```python
from build123d import *

# Parameters (mm, degrees)
F0_R     = 2.032
F1_DEPTH = 19.05
F3_DEPTH = 304.8


with BuildPart() as f1:
    # F0 (on Top) → F1 (new body)
    with BuildSketch(Plane.XY):
        with BuildLine():
            Line((111.125, 152.4), (-69.85, 152.4))
            ThreePointArc((-69.85, 152.4), (-81.939168, 123.214168), (-111.125, 111.125))
            Line((-111.125, 111.125), (-111.125, -111.125))
            ThreePointArc((-111.125, -111.125), (-81.939168, -123.214168), (-69.85, -152.4))
            Line((-69.85, -152.4), (111.125, -152.4))
            Line((111.125, -152.4), (111.125, 152.4))
        make_face()
        with Locations((-63.5, -101.6)):
            Circle(F0_R, mode=Mode.SUBTRACT)
        with Locations((9.525, -127)):
            Circle(F0_R, mode=Mode.SUBTRACT)
        with Locations((77.7875, -101.6)):
            Circle(F0_R, mode=Mode.SUBTRACT)
        with Locations((-63.5, 101.6)):
            Circle(F0_R, mode=Mode.SUBTRACT)
        with Locations((9.525, 127)):
            Circle(F0_R, mode=Mode.SUBTRACT)
        with Locations((77.7875, 101.6)):
            Circle(F0_R, mode=Mode.SUBTRACT)
    extrude(amount=F1_DEPTH)

    # F2 (on face) → F3 (cut, through all)
    with BuildSketch(Plane.XZ.offset(152.4)):
        Polygon((111.125, 0), (111.125, 19.05), (104.191367, 19.05), align=None)
    extrude(amount=-F3_DEPTH, mode=Mode.SUBTRACT)


solid = f1.part
```
Check sheet for the modelled part. Datum: model origin and axes. Units: mm. Give positions to 0.01 mm unless a question says otherwise; leave off trailing zeros. Loops run counter-clockwise (first coordinate to the right, second up) from the corner with the lowest first, then second, coordinate; pieces in that order, holes last. Notation, with made-up numbers: M -8.5,6 L -2.5,6 A22 cw -2.5,39 Z; hole C 48,62 d1. An arc over 180 degrees is marked long. Answer as CSV lines item,"result".
Item 1: Depth check by flat-ended pin: pin 1 Ø3.5 at (x, y) = (77.79, -101.6) entering from -Z; pin 2 Ø3 at (y, z) = (-48.5, 13) entering from +X; pin 3 Ø4 at (y, z) = (40, 13) entering from +X. Enter the tip coordinate at first touch or a pass-through.
Reply:
pin 1,"through"
pin 2,"x = 106.94"
pin 3,"x = 107.12"
Item 2: Sectioned sample at C-C, the plane x = -97. Enter the section's corners in (y, z), then the cut area to 3 significant figures.
Reply:
outline,"M -113.62,0 L 113.62,0 L 113.62,19.05 L -113.62,19.05 Z"
area,"4,330 mm^2"
Item 3: Scan lines: L1, parallel to Y at x = -63.5, z = 12.5; L2, parallel to Y at x = -76.5, z = 6; L3, parallel to Y at x = -95, z = 16.25. Record each from-to range of solid material in increasing order.
Reply:
L1,"-152.4 to -103.63, -99.57 to 99.57, 103.63 to 152.4"
L2,"-129.93 to 129.93"
L3,"-114.41 to 114.41"
Item 4: Sectioned sample at A-A, the plane z = 15.75. State how many separate pieces and enclosed holes the cut face has, then the cut area to 3 significant figures.
Reply:
separate pieces,"1"
enclosed holes,"6"
area,"63,200 mm^2"
Item 5: Sectioned sample at B-B, the plane y = -70.5. Enter the section's corners in (x, z) (3 decimals), then the cut area to 3 significant figures.
Reply:
outline,"M -111.125,0 L 111.125,0 L 104.191,19.05 L -111.125,19.05 Z"
area,"4,170 mm^2"
